Answer from the drawing. Dimensions are ordinates in mm from the lowest x, y and z of the part. Coordinates: 2 decimals unless noted, no trailing zeros. Write each loop counter-clockwise with the first axis right and the second up, starting at its lowest first coordinate (ties: lowest second). Pieces come first, ordered by that corner, then holes.
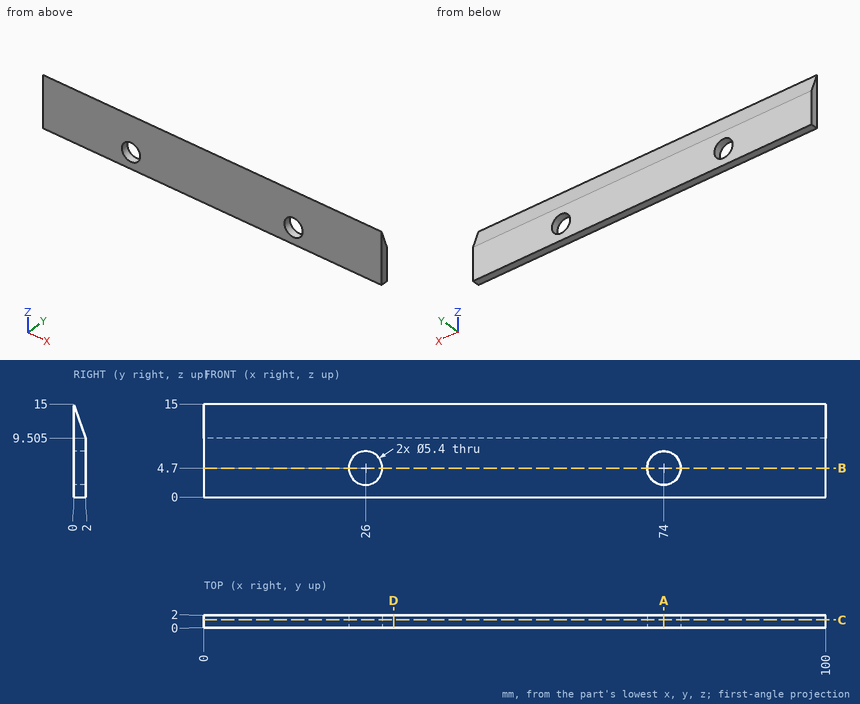
(1) Section C-C, the plane y = 1.25 is taken. Write down the section's boundary in (x, z), plus the area to 3 significant figures.
(2) Section A-A, the plane x = 74 is taken. Write down the section's boundary in (y, z) (3 decimals), plus the area to 3 significant figures.
(3) Section B-B, the plane z = 4.7 is taken. Write down the section's boundary in (x, y), plus the area to 3 significant figures.
(4) Find the intervals of material crossed by probe 1 along X at (y, z) = (1.5, 4.7); probe 2 along X at (y, z) = (0.65, 3.75); probe 3 along Y at (x, z) = (79.5, 9.75), in increasing order.
(5) Section D-D, the plane x = 30.5 is taken. Write down the section's boundary in (y, z) (3 decimals).
(6) Each of these flat-tipped pins is pushed along its axis until it touches: pin 1 (1 mm diameter, centred on x = 57, y = 0.5, fed in from -Z); pin 2 (3 mm diameter, centred on x = 74, z = 4.7, fed in from -Y). Where does it stop, or does it pass through?
Solution:
1. outline: (0, 0) - (100, 0) - (100, 11.57) - (0, 11.57) - close; hole circle Ø5.4 at (26, 4.7); hole circle Ø5.4 at (74, 4.7)
1. area: 1,110 mm2
2. outline: (0, 0) - (2, 0) - (2, 2) - (0, 2) - close; (0, 7.4) - (2, 7.4) - (2, 9.505) - (0, 15) - close
2. area: 13.7 mm2
3. outline: (0, 0) - (23.3, 0) - (23.3, 2) - (0, 2) - close; (28.7, 0) - (71.3, 0) - (71.3, 2) - (28.7, 2) - close; (76.7, 0) - (100, 0) - (100, 2) - (76.7, 2) - close
3. area: 178 mm2
4. probe 1: x = 0 to 23.3, 28.7 to 71.3, 76.7 to 100
4. probe 2: x = 0 to 23.47, 28.53 to 71.47, 76.53 to 100
4. probe 3: y = 0 to 1.91
5. outline: (0, 0) - (2, 0) - (2, 9.505) - (0, 15) - close
6. pin 1: stops at z = 0
6. pin 2: passes through
